Could you check a few things on this model? Use its own coordinates, in mm. Coordinates: 2 decimals unless noted, no trailing zeros. Loops run counter-clockwise (first coordinate to the right, second up) from the corner with the lowest first, then second, coordinate; pieces in that order, holes last.
1) Will these pins go through, and if not, where does the flat tip stop? P1, Ø25, axis at x = -4.5, y = -37, coming from the +Z side; P2, Ø3, axis at x = -17, y = -12.5, coming from the +Z side; P3, Ø6, axis at x = -5.5, y = -20.5, coming from the +Z side.
2) Imagine slicing it at A-A on x = 10. Please give me the cut outline in (y, z).
3) Thinking about a two-plate mould opening in X: for faces 1 (the face through (-37.5, 2, 979)), 2 (the face through (-0.525, -0.234, 1960.461)), 3 (the face through (37.5, 2, 979)), which applies, released by +X, released by -X, zero draft, split by the parting line, or undercut?
4) If I drill on line 1 along Z through (x, y) = (-24, 14.5); line 2 along Z through (x, y) = (-29, -32.5); line 3 along Y through (x, z) = (-22, 1882.5), over which ranges is the centre line in solid material (lowest first)?
```python
from build123d import *

# Parameters (mm, degrees)
F0_W     = 75
F0_H     = 87.5
F1_DEPTH = 2000
F2_R     = 5
F3_W     = 5
F3_H     = 51
F4_DEPTH = 75.001
F5_R     = 2


# Not quite as in the source:
# - a feature names something its author has since deleted; it is built from what else it names


with BuildPart() as f1:
    # F0 (on Top) → F1 (new body)
    with BuildSketch(Plane.XY):
        Rectangle(F0_W, F0_H)
    extrude(amount=F1_DEPTH)

    # F2
    f2_edges = [f1.edges().sort_by_distance(p)[0] for p in [
        (-37.5, -43.75, 1000),
        (37.5, -43.75, 1000),
    ]]
    fillet(f2_edges, radius=F2_R)

    # F3 (on face) → F4 (cut, through all)
    with BuildSketch(Plane(origin=(-37.5, 0, 0), x_dir=(0, -1, 0), z_dir=(-1, 0, 0))):
        with BuildLine():
            Line((-28.8070795286, 1845.5327422672), (-16.605275544, 1985))
            Line((-16.605275544, 1985), (-1.7898756174, 1983.7038204608))
            ThreePointArc((-1.7898756174, 1983.7038204608), (0.4221879267, 1960.172410035), (21.25, 1949))
            Line((21.25, 1949), (38.75, 1949))
            Line((38.75, 1949), (38.75, 2000))
            Line((38.75, 2000), (-43.75, 2000))
            Line((-43.75, 2000), (-43.75, 1846.8400784084))
            Line((-43.75, 1846.8400784084), (-28.8070795286, 1845.5327422672))
        make_face()
        with Locations((41.25, 1974.5)):
            Rectangle(F3_W, F3_H)
    extrude(amount=-F4_DEPTH, mode=Mode.SUBTRACT)

    # F5
    f5_edges = [f1.edges().sort_by_distance(p)[0] for p in [
        (0, 16.605276, 1985),
        (0, 28.80708, 1845.532742),
    ]]
    fillet(f5_edges, radius=F5_R)


solid = f1.part
```
Filled in:
1. P1: stops at z = 1949
1. P2: stops at z = 1951.2
1. P3: stops at z = 1949.28
2. outline: (-43.75, 0) - (43.75, 0) - (43.75, 1846.84) - (30.8, 1845.71) arc R2 cw to (28.63, 1847.53) - (16.78, 1983.01) arc R2 ccw to (14.61, 1984.83) - (1.79, 1983.7) arc R25 cw to (-21.25, 1949) - (-43.75, 1949) - close
3. face 1: released by -X
3. face 2: zero draft
3. face 3: released by +X
4. line 1: z = 0 to 1984.82
4. line 2: z = 0 to 1949
4. line 3: y = -43.75 to 25.57
